from build123d import *

# Parameters (mm, degrees)
SKETCH3_R           = 5
BOSS_EXTRUDE2_DEPTH = 5
BOSS_EXTRUDE3_START = 2
SKETCH4_R           = 5
BOSS_EXTRUDE3_DEPTH = 2
SKETCH5_W           = 3.7592
SKETCH5_H           = 2
CUT_EXTRUDE2_DEPTH  = 0.5
SKETCH6_W           = 3.7592
SKETCH6_H           = 2
CUT_EXTRUDE3_DEPTH  = 0.5
SKETCH7_W           = 2
SKETCH7_H           = 4.7592
CUT_EXTRUDE4_DEPTH  = 0.5
SKETCH8_W           = 2
SKETCH8_H           = 4.7592
CUT_EXTRUDE5_DEPTH  = 0.5
FILLET1_R           = 1


with BuildPart() as part:
    # Sketch3 → Boss-Extrude2 (new body)
    with BuildSketch(Plane.XY.offset(2.9718)):
        with Locations((30.41838411, -58.09837557)):
            Circle(SKETCH3_R)
    extrude(amount=BOSS_EXTRUDE2_DEPTH)

    # Sketch4 → Boss-Extrude3 (add)
    with BuildSketch(Plane(origin=(0, 0, 2.9718), x_dir=(-1, 0, 0), z_dir=(0, 0, -1)).offset(BOSS_EXTRUDE3_START)):
        with Locations((-30.41838411, -58.09837557)):
            Circle(SKETCH4_R)
        Polygon((-30.505343509, -60.755108598), (-33.075117138, -58.011416171), (-30.331424712, -55.441642541), (-27.761651082, -58.185334968), align=None, mode=Mode.SUBTRACT)
    extrude(amount=-BOSS_EXTRUDE3_DEPTH)

    # Sketch5 → Cut-Extrude2 (cut)
    with BuildSketch(Plane(origin=(-13.487510975, -14.400327439, 0), x_dir=(0.7298607220838652, -0.6835958794194263, 0), z_dir=(-0.6835958794194263, -0.7298607220838652, 0))):
        with Locations((61.916993932, 1.9718)):
            Rectangle(SKETCH5_W, SKETCH5_H)
    extrude(amount=-CUT_EXTRUDE2_DEPTH, mode=Mode.SUBTRACT)

    # Sketch6 → Cut-Extrude3 (cut)
    with BuildSketch(Plane(origin=(-16.057284605, -17.144019865, 0), x_dir=(0.7298607220838642, -0.6835958794194275, 0), z_dir=(0.6835958794194275, 0.7298607220838642, 0))):
        with Locations((61.916993932, -1.9718)):
            Rectangle(SKETCH6_W, SKETCH6_H)
    extrude(amount=-CUT_EXTRUDE3_DEPTH, mode=Mode.SUBTRACT)

    # Sketch7 → Cut-Extrude4 (cut)
    with BuildSketch(Plane(origin=(43.818935687, -41.041315103, 0), x_dir=(0, 0, -1), z_dir=(0.7298607220838652, -0.6835958794194263, 0))):
        with Locations((-1.9718, -21.609840309)):
            Rectangle(SKETCH7_W, SKETCH7_H)
    extrude(amount=-CUT_EXTRUDE4_DEPTH, mode=Mode.SUBTRACT)

    # Sketch8 → Cut-Extrude5 (cut)
    with BuildSketch(Plane(origin=(46.562628114, -43.611088733, 0), x_dir=(0, 0, 1), z_dir=(-0.7298607220838662, 0.6835958794194253, 0))):
        with Locations((1.9718, -21.609840309)):
            Rectangle(SKETCH8_W, SKETCH8_H)
    extrude(amount=-CUT_EXTRUDE5_DEPTH, mode=Mode.SUBTRACT)

    # Fillet1
    fillet1_edges = [part.edges().sort_by_distance(p)[0] for p in [
        (25.41838411, -58.09837557, 7.9718),
    ]]
    fillet(fillet1_edges, radius=FILLET1_R)


solid = part.part
The listing builds one solid part. Answer for the finished solid, in the listing's coordinates (mm). A direction names the side the tool comes from. Give positions to 0.01 mm unless a question says otherwise; leave off trailing zeros. Write each loop counter-clockwise with the first axis right and the second up, starting at its lowest first coordinate (ties: lowest second). Pieces come first, ordered by that corner, then holes. Notation, with made-up numbers: (-20.75, 15) -> (11.25, 15) arc R20 cw to (11.25, 29) -> close; hole circle Ø3 at (-39, 87.25). An arc over 180 degrees is marked (long way). Use a Markdown table: item, result.
(1) Find the intervals of material crossed by probe 1 along X at (y, z) = (-58.25, 4.5); probe 2 along X at (y, z) = (-57.75, 2.5); probe 3 along Z at (x, y) = (29.25, -56.5), in increasing order. Write a range as from..to.
Return value:
| item | result |
|---|---|
| probe 1 | 25.42..35.42 |
| probe 2 | 25.43..27.48, 33.53..35.41 |
| probe 3 | 2.97..7.97 |
(2) For faces 3 (the flat face through (32.18, -59.7, 1.96)), 4 (the flat face through (30, -58, 7.972)), determine the directions among +Z, -Z, +X, -X, +Y, -Y from which every point of the face is accessible in a straight line to the end or side of a thin tool.
Return value:
| item | result |
|---|---|
| face 3 | -Z |
| face 4 | +Z, +X, -X, +Y, -Y |
(3) Flat-ended cylindrical pins translate along their axes: P1, Ø3, axis at x = 28.5, y = -59.5, coming from the -Z side; P2, Ø1.5, axis at x = 27, y = -61.5, coming from the +Z side; P3, Ø0.9, axis at x = 31, y = -56.5, coming from the -Z side; P4, Ø1.5, axis at x = 32.5, z = 5, coming from the +Y side. Find the tip coordinate at first contact, or state that the pin passes through.
Return value:
| item | result |
|---|---|
| P1 | z = 0.97 |
| P2 | z = 7.97 |
| P3 | z = 2.97 |
| P4 | y = -53.28 |
(4) Section A-A, the plane z = 2.5 is taken. Determine the outline of the cut face in (x, y).
Return value:
| item | result |
|---|---|
| outline | circle Ø10 at (30.42, -58.1); hole (27.05, -58.21) -> (30.53, -61.46) -> (33.78, -57.99) -> (30.31, -54.73) -> close |
(5) Determine the mould class of faces 1 (the flat face through (28.7, -56.45, 1.99)), 2 (the flat face through (33, -57, 0.972)) for opening direction X: released by +X, released by -X, zero draft, split by the parting line, or undercut.
Return value:
| item | result |
|---|---|
| face 1 | undercut |
| face 2 | zero draft |
(6) Section B-B, the plane z = 6.5 is taken. Determine the outline of the cut face in (x, y).
Return value:
| item | result |
|---|---|
| outline | circle Ø10 at (30.42, -58.1) |
(7) Section C-C, the plane z = 7.5 is taken. Determine the outline of the cut face in (x, y).
Return value:
| item | result |
|---|---|
| outline | circle Ø9.7 at (30.42, -58.1) |
